Geometry: see drawing. Coordinates: mm, zero at the bounding-box minimum. A direction names the side the tool comes from. Coordinates: 2 decimals unless noted, no trailing zeros. Loops run counter-clockwise (first coordinate to the right, second up) from the corner with the lowest first, then second, coordinate; pieces in that order, holes last. Notation, with made-up numbers: (-14.75, 8.5) - (42.25, 8.5) arc R11 cw to (42.25, 19.5) - close; hole circle Ø11 at (-37.5, -9.5). An arc over 180 degrees is marked (long way). Use one line per item in the form item = value.
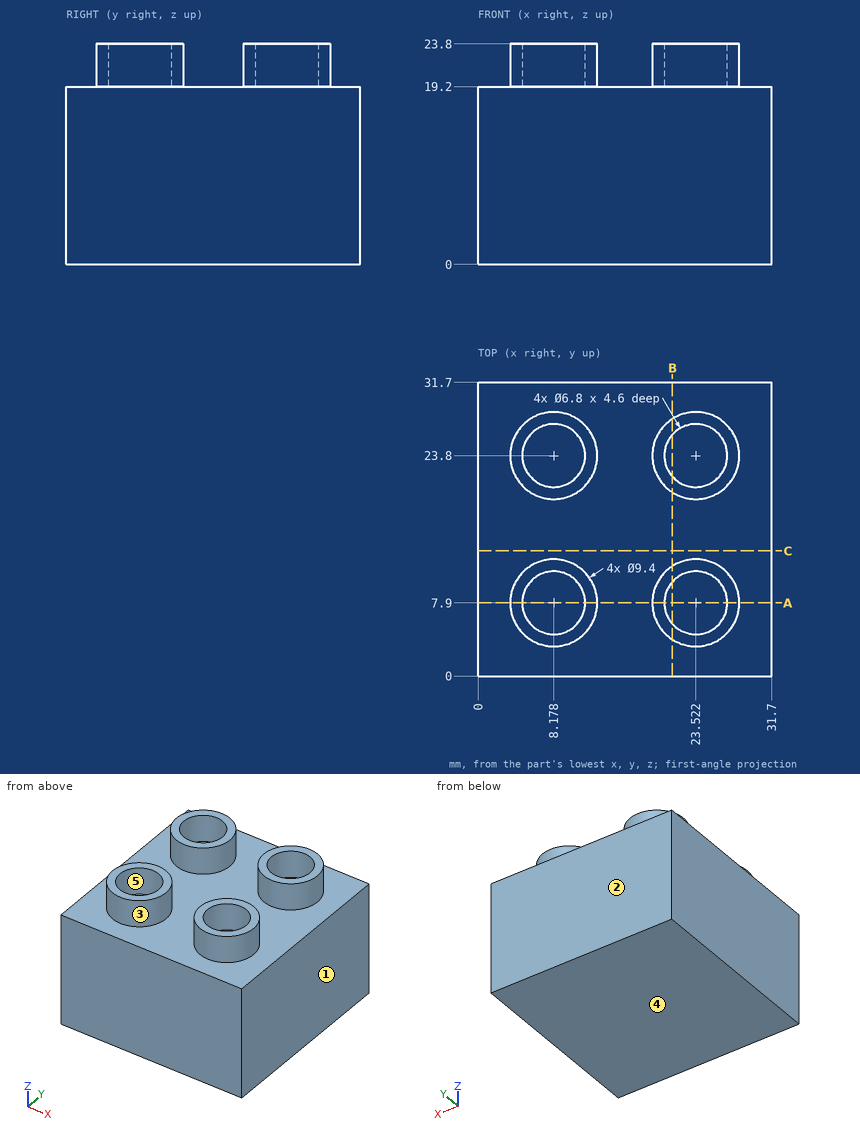
Q1. Pull-direction query (Y, two-part tool) for the marked faces 1, 2 and 3; classes: pulls with the +Y half, pulls with the -Y half, needs draft (parallel to the pull), parting line crosses it, or undercut.
Check values:
face_1 = needs draft
face_2 = pulls with the +Y half
face_3 = undercut
Q2. First-contact query: P1, Ø4, axis at x = 8.18, y = 7.9, coming from the +Z side. Flat tip, straight axial feed; report the tip coordinate or a pass-through.
Check values:
P1 = 19.2
Q3. Ray query, line 1 along Y through (x, z) = (8.5, 21.25) (1 decimal); line 2 along Y through (x, z) = (7.5, 21.5); line 3 along Z through (x, y) = (16, 18). Return the intervals inside material, ascending. Write a range as [from, to].
Check values:
line_1 = [3.2, 4.5], [11.3, 12.6], [19.1, 20.4], [27.2, 28.5]
line_2 = [3.25, 4.57], [11.23, 12.55], [19.15, 20.47], [27.13, 28.45]
line_3 = [0, 19.2]
Q4. Set-up query: the marked faces 4 and 5. Return all of +Z, -Z, +X, -X, +Y, -Y with unobstructed straight access to the full face (end or side cutting, diameter ignored); none if empty.
Check values:
face_4 = -Z, +X, -X, +Y, -Y
face_5 = +Z
Q5. Cut plane B-B, the plane x = 21. Return loops of the section in (y, z), then the cut area to 3 significant figures.
Check values:
outline = (0, 0) - (31.7, 0) - (31.7, 19.2) - (27.77, 19.2) - (27.77, 23.8) - (26.08, 23.8) - (26.08, 19.2) - (21.52, 19.2) - (21.52, 23.8) - (19.83, 23.8) - (19.83, 19.2) - (11.87, 19.2) - (11.87, 23.8) - (10.18, 23.8) - (10.18, 19.2) - (5.62, 19.2) - (5.62, 23.8) - (3.93, 23.8) - (3.93, 19.2) - (0, 19.2) - close
area = 640 mm²
Q6. Cut plane A-A, the plane y = 7.9. Return loops of the section in (x, z).
Check values:
outline = (0, 0) - (31.7, 0) - (31.7, 19.2) - (28.22, 19.2) - (28.22, 23.8) - (26.92, 23.8) - (26.92, 19.2) - (20.12, 19.2) - (20.12, 23.8) - (18.82, 23.8) - (18.82, 19.2) - (12.88, 19.2) - (12.88, 23.8) - (11.58, 23.8) - (11.58, 19.2) - (4.78, 19.2) - (4.78, 23.8) - (3.48, 23.8) - (3.48, 19.2) - (0, 19.2) - close
Q7. Cut plane C-C, the plane y = 13.5. Return loops of the section in (x, z), then the cut area to 3 significant figures.
Check values:
outline = (0, 0) - (31.7, 0) - (31.7, 19.2) - (0, 19.2) - close
area = 609 mm²
